Design review of the part shown in the three views and the two pictorial views. Dimensions are in mm from the part's minimum x, y and z. A direction names the side the tool comes from. Round coordinates to 2 decimals unless told otherwise and drop trailing zeros. Order: outer loops, then holes, each group sorted by start corner. A loop starts at its lowest first (then second) coordinate and runs counter-clockwise, first axis right, second up.
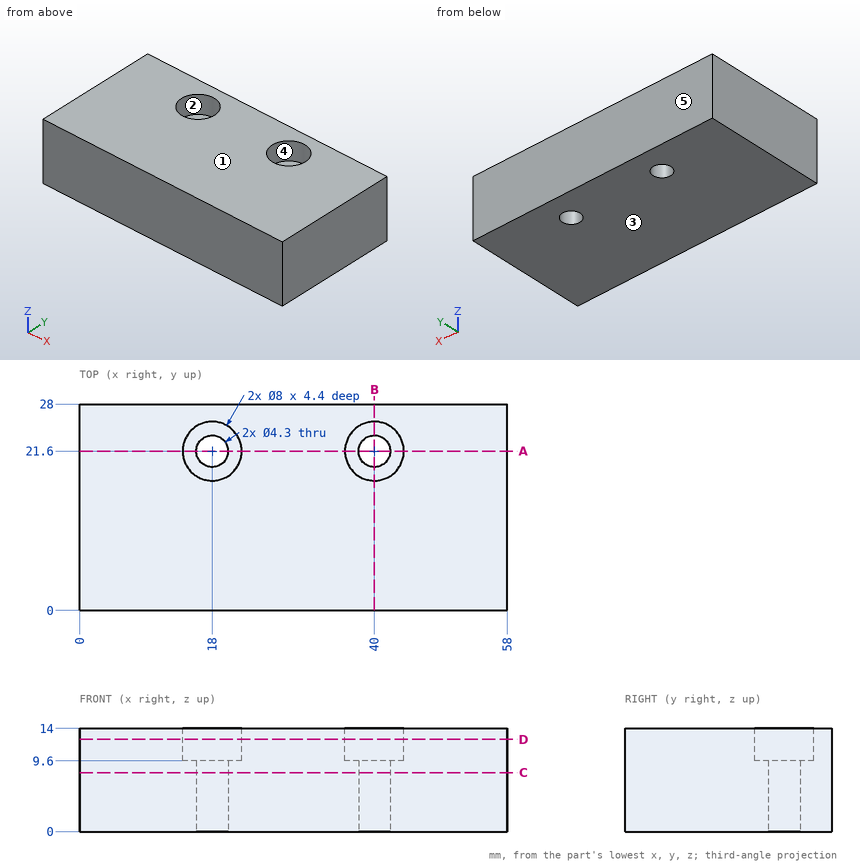
(1) Draft analysis for pull direction Y (two halves, no side actions). For the marked faces 3, 4 and 5, state which applies: pulls with the +Y half, pulls with the -Y half, needs draft (parallel to the pull), parting line crosses it, or undercut.
Data:
face 3: needs draft
face 4: undercut
face 5: pulls with the +Y half
(2) Consider section C-C (z = 8). Write out the cut boundary in (x, y), and give its area (3 significant figures).
Data:
outline: (0, 0) - (58, 0) - (58, 28) - (0, 28) - close; hole circle Ø4.3 at (18, 21.6); hole circle Ø4.3 at (40, 21.6)
area: 1,590 mm2
(3) Insertion check: pin 1 (1 mm diameter, centred on x = 19.5, y = 20, fed in from +Z). The pin has a flat end and moves straight along its axis. Give the tip position at first contact, or say it passes through.
Data:
pin 1: stops at z = 9.6
(4) For the marked faces 1 and 2, list the 3-axis set-ups (+Z, -Z, +X, -X, +Y, -Y) from which the entire face can be reached by the end or side of a thin tool; tool diameter is ignored.
Data:
face 1: +Z, +X, -X, +Y, -Y
face 2: +Z
(5) To check wall thickness, follow probe 1 along Y at (x, z) = (18, 10.65); probe 2 along X at (y, z) = (23, 10.75); probe 3 along Y at (x, z) = (18, 8.75). State the ranges of each line that lie inside material, in increasing order.
Data:
probe 1: y = 0 to 17.6, 25.6 to 28
probe 2: x = 0 to 14.25, 21.75 to 36.25, 43.75 to 58
probe 3: y = 0 to 19.45, 23.75 to 28
(6) Consider section D-D (z = 12.5). Write out the cut boundary in (x, y), and give its area (3 significant figures).
Data:
outline: (0, 0) - (58, 0) - (58, 28) - (0, 28) - close; hole circle Ø8 at (18, 21.6); hole circle Ø8 at (40, 21.6)
area: 1,520 mm2
(7) Consider section B-B (x = 40). Write out the cut boundary in (y, z).
Data:
outline: (0, 0) - (19.45, 0) - (19.45, 9.6) - (17.6, 9.6) - (17.6, 14) - (0, 14) - close; (23.75, 0) - (28, 0) - (28, 14) - (25.6, 14) - (25.6, 9.6) - (23.75, 9.6) - close
(8) Consider section A-A (y = 21.6). Write out the cut boundary in (x, z), and give its area (3 significant figures).
Data:
outline: (0, 0) - (15.85, 0) - (15.85, 9.6) - (14, 9.6) - (14, 14) - (0, 14) - close; (20.15, 0) - (37.85, 0) - (37.85, 9.6) - (36, 9.6) - (36, 14) - (22, 14) - (22, 9.6) - (20.15, 9.6) - close; (42.15, 0) - (58, 0) - (58, 14) - (44, 14) - (44, 9.6) - (42.15, 9.6) - close
area: 659 mm2
